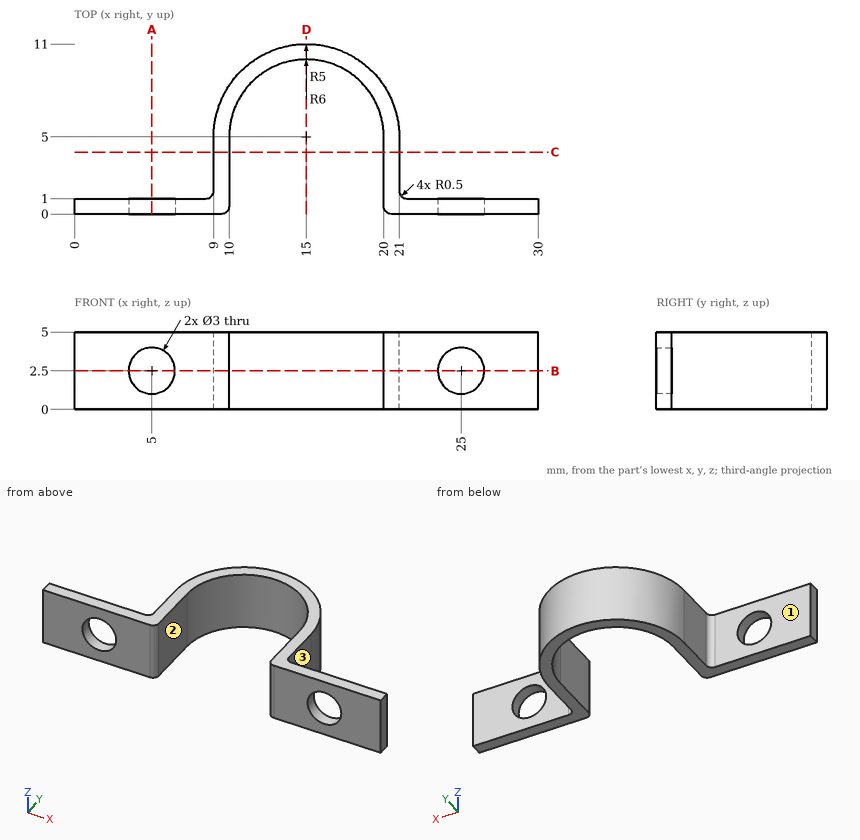
Here's the drawing with two shaded views (mm, measured from the low corner). I have some questions. A direction names the side the tool comes from. Coordinates: 2 decimals unless noted, no trailing zeros. Write each loop counter-clockwise with the first axis right and the second up, starting at its lowest first coordinate (ties: lowest second). Pieces come first, ordered by that corner, then holes. Notation, with made-up numbers: M 57,8 L 81,8 A23 ccw 81,27 Z; hole C 15,2 d5. An arc over 180 degrees is marked long. Answer as CSV lines item,"result". Start each with the question number.
1) I want a section at B-B, the plane z = 2.5. Please give me the cut outline in (x, y).
2) I want a section at C-C, the plane y = 4. Please give me the cut outline in (x, z), and give its area (3 significant figures).
3) Please list where these lines run through material, in increasing order: line 1 (X direction, y = 0.7, z = 2.5); line 2 (X direction, y = 5, z = 3.05); line 3 (Z direction, x = 5, y = 0.75). Write a range as from..to.
4) For the marked faces 1, 2 and 3, which set-ups out of +Z, -Z, +X, -X, +Y, -Y let a thin tool reach every point of the face, with its end or its side?
5) I want a section at A-A, the plane x = 5. Please give me the cut outline in (y, z).
6) I want a section at D-D, the plane x = 15. Please give me the cut outline in (y, z).
7) For P1, Ø2, axis at x = 17.5, z = 4.5, coming from the +Y side; P2, Ø1.8, axis at y = 3.5, z = 3.5, coming from the +X side; P3, Ø1.8, axis at y = 3.5, z = 1.5, coming from the -X side, each with a flat end and sliding along its axis, tell me the tip position at first contact or that it passes through.
Data:
1,outline,"M 0,0 L 3.5,0 L 3.5,1 L 0,1 Z; M 6.5,0 L 9.5,0 A0.5 ccw 10,0.5 L 10,5 A5 cw 20,5 L 20,0.5 A0.5 ccw 20.5,0 L 23.5,0 L 23.5,1 L 21.5,1 A0.5 cw 21,1.5 L 21,5 A6 ccw 9,5 L 9,1.5 A0.5 cw 8.5,1 L 6.5,1 Z; M 26.5,0 L 30,0 L 30,1 L 26.5,1 Z"
2,outline,"M 9,0 L 10,0 L 10,5 L 9,5 Z; M 20,0 L 21,0 L 21,5 L 20,5 Z"
2,area,"10.0 mm^2"
3,line 1,"x = 0..3.5, 6.5..10, 20..23.5, 26.5..30"
3,line 2,"x = 9..10, 20..21"
3,line 3,"z = 0..1, 4..5"
4,face 1,"+Z, -Z, -X, +Y"
4,face 2,"+Z, -Z, -Y"
4,face 3,"+Z, -Z, +X, +Y"
5,outline,"M 0,0 L 1,0 L 1,1 L 0,1 Z; M 0,4 L 1,4 L 1,5 L 0,5 Z"
6,outline,"M 10,0 L 11,0 L 11,5 L 10,5 Z"
7,P1,"stops at y = 10.81"
7,P2,"stops at x = 21"
7,P3,"stops at x = 9"
